Autodesk Inventor part; units mm, degrees
ref_plane "YZ Plane" through (0, 0, 0) normal (1, 0, 0) x (0, 1, 0)
ref_plane "XZ Plane" through (0, 0, 0) normal (0, 1, 0) x (-1, 0, 0)
ref_plane "XY Plane" through (0, 0, 0) normal (0, 0, 1) x (1, 0, 0)
sketch "Esquisse1" plane through (0, 0, 0) normal (0, 1, 0) x (-1, 0, 0)
  circle A0 centre (0, 0) radius 15
  dimension "d0" = 30
extrude "Extrusion1" add sketch "Esquisse1" along normal blind 6
fillet "Congé1" radius 2 2 edges at (15, 6, 0) (15, 0, 0)
sketch "Esquisse2" plane through (0, 6, 0) normal (0, 1, 0) x (1, 0, 0)
  circle A0 centre (0, 0) radius 12.5
  dimension "d6" = 25
extrude "Extrusion2" cut sketch "Esquisse2" against normal blind 10
thread "Filetage2"
properties part number "Anneau inf"
Verification items for the finished model (mm, model axes). Coordinates: 2 decimals unless noted, no trailing zeros. Write each loop counter-clockwise with the first axis right and the second up, starting at its lowest first coordinate (ties: lowest second). Pieces come first, ordered by that corner, then holes. Notation, with made-up numbers: (11, 32.5) -> (64, 32.5) arc R29 cw to (64, 62.5) -> close; hole circle Ø3 at (-13.5, 58.25). An arc over 180 degrees is marked (long way). One line per item, written item: value. Start each with the question number.
Q1. Cross-section at B-B on x = 0. Enter the section's corners in (y, z), and give its area (3 significant figures).
Q2. Cross-section at C-C on y = 3.45. Enter the section's corners in (x, z).
Q3. Thickness scan on L1, parallel to Z at x = 0, y = 2.45; L2, parallel to X at y = 5.35, z = -0.25; L3, parallel to X at y = 1.1, z = -1.5. Record the ranges inside material, lowest first. Write a range as from..to.
Q4. Cross-section at A-A on z = 0. Enter the section's corners in (x, y), and give its area (3 significant figures).
Q5. Cross-section at D-D on y = 1.6. Enter the section's corners in (x, z), and give its area (3 significant figures).
Q6. Mould release check, pull along Z, two halves, no side actions. Record for faces 1 (the cylindrical face through (14.985, 2.986, -0.66)), 2 (the cylindrical face through (11.923, 3.042, -3.755)), 3 (the flat face through (6.8, 0, 10.7)): pulls with the +Z half, pulls with the -Z half, needs draft (parallel to the pull), parting line crosses it, or undercut.
Checked values:
1. outline: (0, -13) arc R2 ccw to (2, -15) -> (4, -15) arc R2 ccw to (6, -13) -> (6, -12.5) -> (0, -12.5) -> close; (0, 12.5) -> (6, 12.5) -> (6, 13) arc R2 ccw to (4, 15) -> (2, 15) arc R2 ccw to (0, 13) -> close
1. area: 26.6 mm²
2. outline: circle Ø30 at (0, 0); hole circle Ø25 at (0, 0)
3. L1: z = -15..-12.5, 12.5..15
3. L2: x = -14.47..-12.5, 12.5..14.47
3. L3: x = -14.71..-12.41, 12.41..14.71
4. outline: (-15, 2) arc R2 ccw to (-13, 0) -> (-12.5, 0) -> (-12.5, 6) -> (-13, 6) arc R2 ccw to (-15, 4) -> close; (12.5, 0) -> (13, 0) arc R2 ccw to (15, 2) -> (15, 4) arc R2 ccw to (13, 6) -> (12.5, 6) -> close
4. area: 26.6 mm²
5. outline: circle Ø29.92 at (0, 0); hole circle Ø25 at (0, 0)
5. area: 212 mm²
6. face 1: parting line crosses it
6. face 2: undercut
6. face 3: needs draft
